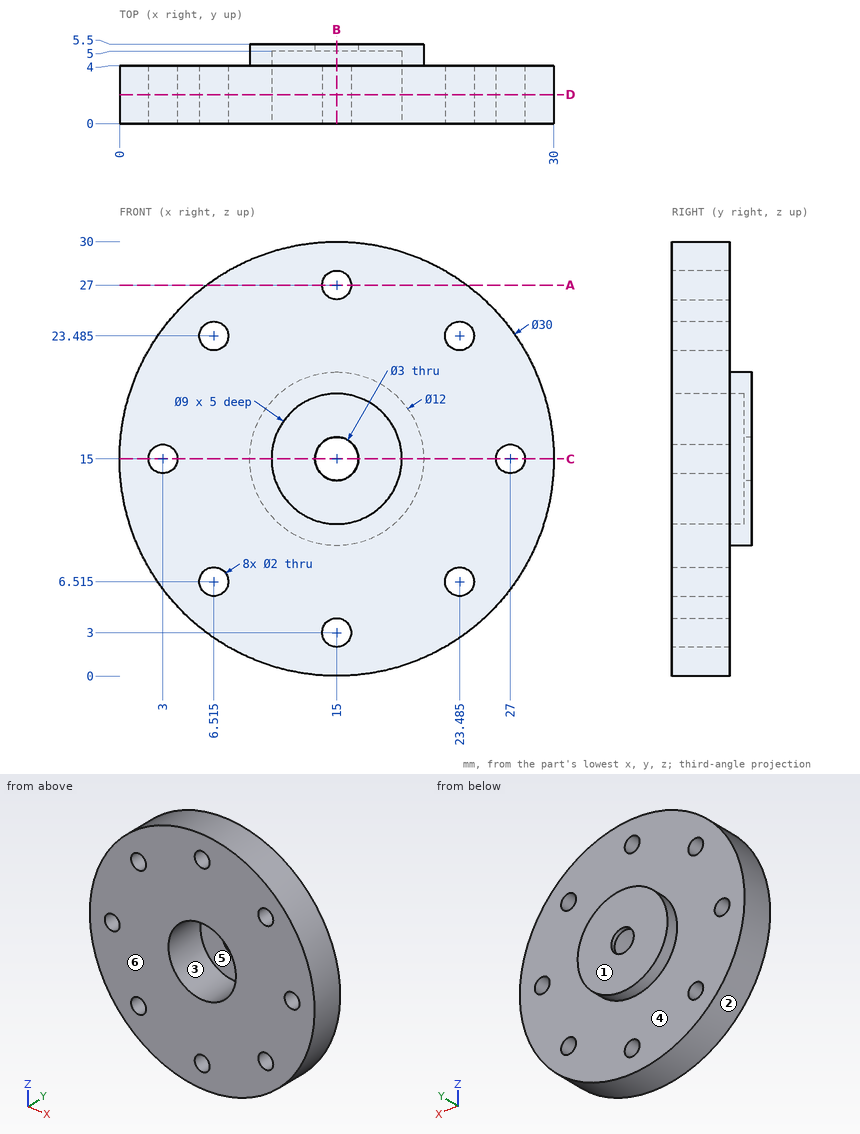
The figure shows three views and two pictorial views of one solid part (mm, origin at its lowest corner). Answer the questions. A direction names the side the tool comes from. Give positions to 0.01 mm unless a question says otherwise; leave off trailing zeros. Write each loop counter-clockwise with the first axis right and the second up, starting at its lowest first coordinate (ties: lowest second). Pieces come first, ordered by that corner, then holes. Notation, with made-up numbers: (6.5, 79.5) - (22.5, 79.5) arc R21 cw to (22.5, 112.5) - close; hole circle Ø6 at (19.5, -13). An arc over 180 degrees is marked (long way). Use one line per item in the form item = value. Start each with the question number.
1) Flat-ended cylindrical pins translate along their axes: pin 1 Ø1.6 at (x, z) = (6.51, 23.49) entering from -Y; pin 2 Ø2.5 at (x, z) = (15, 3) entering from +Y; pin 3 Ø7 at (x, z) = (15, 15) entering from -Y; pin 4 Ø3 at (y, z) = (1.5, 7) entering from -X. Find the tip coordinate at first contact, or state that the pin passes through.
2) Find section B-B on x = 15. Determine the outline of the cut face in (y, z).
3) Find section C-C on z = 15. Determine the outline of the cut face in (x, y).
4) The mould has two halves that part along Z. Classify the marked faces 1, 2 and 3: pulls with the +Z half, pulls with the -Z half, needs draft (parallel to the pull), parting line crosses it, or undercut.
5) Consider line 1 along X through (y, z) = (2, 15); line 2 along Z through (x, y) = (24, 2.85); line 3 along Z through (x, y) = (23.5, 3.1) (1 decimal). Determine where each line is inside the solid, lowest interval first. Write a range as from..to.
6) A tool of negligible diameter and unlimited length cuts with its end or side. For the marked faces 4, 5 and 6, from which of +Z, -Z, +X, -X, +Y, -Y can it reach the whole face along a straight path? Write none if from no direction.
7) Find section A-A on z = 27. Determine the outline of the cut face in (x, y).
8) Find section D-D on y = 2. Count the separate pieces of the cut face and the enclosed holes in it, plus the area to 3 significant figures.
Geometry results:
q1.pin_1 = through
q1.pin_2 = 4
q1.pin_3 = 5
q1.pin_4 = 1.48
q2.outline = (0, 0) - (4, 0) - (4, 2) - (0, 2) - close; (0, 4) - (4, 4) - (4, 9) - (5.5, 9) - (5.5, 13.5) - (5, 13.5) - (5, 10.5) - (0, 10.5) - close; (0, 19.5) - (5, 19.5) - (5, 16.5) - (5.5, 16.5) - (5.5, 21) - (4, 21) - (4, 26) - (0, 26) - close; (0, 28) - (4, 28) - (4, 30) - (0, 30) - close
q3.outline = (0, 0) - (2, 0) - (2, 4) - (0, 4) - close; (4, 0) - (10.5, 0) - (10.5, 5) - (13.5, 5) - (13.5, 5.5) - (9, 5.5) - (9, 4) - (4, 4) - close; (16.5, 5) - (19.5, 5) - (19.5, 0) - (26, 0) - (26, 4) - (21, 4) - (21, 5.5) - (16.5, 5.5) - close; (28, 0) - (30, 0) - (30, 4) - (28, 4) - close
q4.face_1 = needs draft
q4.face_2 = parting line crosses it
q4.face_3 = undercut
q5.line_1 = 0..2, 4..10.5, 19.5..26, 28..30
q5.line_2 = 3..5.66, 7.37..22.63, 24.34..27
q5.line_3 = 2.6..5.5, 7.5..22.5, 24.5..27.4
q6.face_4 = +Y
q6.face_5 = -Y
q6.face_6 = +Z, -Z, +X, -X, -Y
q7.outline = (6, 0) - (14, 0) - (14, 4) - (6, 4) - close; (16, 0) - (24, 0) - (24, 4) - (16, 4) - close
q8.separate_pieces = 1
q8.enclosed_holes = 9
q8.area = 618 mm2
